from build123d import *

# Parameters (mm, degrees)
SKETCH1_R           = 3
BOSS_EXTRUDE1_DEPTH = 1.6


with BuildPart() as part:
    # Sketch1 → Boss-Extrude1 (new body)
    with BuildSketch(Plane(origin=(0, 0, 0), x_dir=(1, 0, 0), z_dir=(0, 1, 0))):
        with BuildLine():
            ThreePointArc((95.75, 0), (98.5, 2.75), (101.25, 0))
            Line((101.25, 0), (102, 0))
            Line((102, 0), (102, 11.75))
            ThreePointArc((102, 11.75), (113.75, 23.5), (125.5, 11.75))
            Line((125.5, 11.75), (125.5, 0))
            Line((125.5, 0), (126.25, 0))
            ThreePointArc((126.25, 0), (129, 2.75), (131.75, 0))
            Line((131.75, 0), (145.25, 0))
            ThreePointArc((145.25, 0), (148, 2.75), (150.75, 0))
            Line((150.75, 0), (151.5, 0))
            Line((151.5, 0), (151.5, 11.75))
            ThreePointArc((151.5, 11.75), (163.25, 23.5), (175, 11.75))
            Line((175, 11.75), (175, 0))
            Line((175, 0), (175.75, 0))
            ThreePointArc((175.75, 0), (178.5, 2.75), (181.25, 0))
            Line((181.25, 0), (190, 0))
            Line((190, 0), (184.397294991, 13.35112683))
            ThreePointArc((184.397294991, 13.35112683), (175.255085608, 21.137460938), (176.103062866, 33.116105511))
            Line((176.103062866, 33.116105511), (166.5, 56))
            Line((166.5, 56), (162.25, 56))
            ThreePointArc((162.25, 56), (159.5, 53.25), (156.75, 56))
            Line((156.75, 56), (156, 56))
            Line((156, 56), (156, 44.25))
            ThreePointArc((156, 44.25), (144.25, 32.5), (132.5, 44.25))
            Line((132.5, 44.25), (132.5, 56))
            Line((132.5, 56), (131.75, 56))
            ThreePointArc((131.75, 56), (129, 53.25), (126.25, 56))
            Line((126.25, 56), (106.5, 56))
            Line((106.5, 56), (106.5, 44.25))
            ThreePointArc((106.5, 44.25), (94.75, 32.5), (83, 44.25))
            Line((83, 44.25), (83, 56))
            Line((83, 56), (35, 56))
            Line((35, 56), (28.772512455, 46.036019928))
            ThreePointArc((28.772512455, 46.036019928), (29.720282193, 45.037138056), (30.06501537, 43.704024592))
            ThreePointArc((30.06501537, 43.704024592), (28.648128834, 41.298757768), (25.857518285, 41.372029256))
            Line((25.857518285, 41.372029256), (23.160953678, 37.057525885))
            ThreePointArc((23.160953678, 37.057525885), (27.537926652, 32.444507786), (29.12996714, 26.287947424))
            ThreePointArc((29.12996714, 26.287947424), (22.586527501, 15.179987912), (9.698980602, 15.518368963))
            Line((9.698980602, 15.518368963), (8.612482775, 13.77997244))
            ThreePointArc((8.612482775, 13.77997244), (9.560252513, 12.781090568), (9.90498569, 11.447977104))
            ThreePointArc((9.90498569, 11.447977104), (8.488099154, 9.042710281), (5.697488605, 9.115981768))
            Line((5.697488605, 9.115981768), (0, 0))
            Line((0, 0), (95.75, 0))
        make_face()
        with Locations(Location((92, 11.75, 0), (0, 0, 270))):  # turned: the seam where the file's is
            Circle(SKETCH1_R, mode=Mode.SUBTRACT)
        with Locations(Location((73, 44.25, 0), (0, 0, 270))):  # turned: the seam where the file's is
            Circle(SKETCH1_R, mode=Mode.SUBTRACT)
        with Locations(Location((122.5, 44.25, 0), (0, 0, 270))):  # turned: the seam where the file's is
            Circle(SKETCH1_R, mode=Mode.SUBTRACT)
    extrude(amount=BOSS_EXTRUDE1_DEPTH)


solid = part.part
Verification items for the finished model (mm, model axes). Coordinates: 2 decimals unless noted, no trailing zeros. Order: outer loops, then holes, each group sorted by start corner. A loop starts at its lowest first (then second) coordinate and runs counter-clockwise, first axis right, second up. Notation, with made-up numbers: M 20,-34 L 38,-34 A13 ccw 38,-14 Z; hole C 83,67.5 d2. An arc over 180 degrees is marked long. Write each question's results on one line, items separated by ' | '.
1) Release check for a two-part mould opening along Z. For faces 1 (the face through (89.07, 0.79, -12.4)), 2 (the face through (94, 0, -28)), 3 (the face through (125.474, 0.789, -44.641)), 4 (the face through (187.24, 0.79, -6.58)) record: pulls with the +Z half, pulls with the -Z half, needs draft (parallel to the pull), parting line crosses it, or undercut.
Solved:
face 1: undercut | face 2: needs draft | face 3: undercut | face 4: pulls with the -Z half
2) Scan lines: line 1 along X through (y, z) = (1.15, -37); line 2 along X through (y, z) = (0.1, -44); line 3 along X through (y, z) = (0.35, -3.5). Record each from-to range of solid material in increasing order. Write a range as [from, to].
Solved:
line 1: x = [23.25, 85.5], [104, 135], [153.5, 174.47] | line 2: x = [30.05, 70.01], [75.99, 83], [106.5, 119.51], [125.49, 132.5], [156, 171.54] | line 3: x = [2.19, 102], [125.5, 151.5], [175, 188.53]
3) Gauge pin test, flat ends, axial feed: pin 1 Ø4 at (x, z) = (69, -11.5) entering from -Y; pin 2 Ø0.8 at (y, z) = (1, -3) entering from -X (3 decimals); pin 3 Ø0.8 at (y, z) = (0.5, -49.5) entering from +X; pin 4 Ø0.5 at (y, z) = (0.5, -49) entering from -X. Record the tip position at first contact, or that the pin passes through.
Solved:
pin 1: stops at y = 0 | pin 2: stops at x = 1.625 | pin 3: stops at x = 169.4 | pin 4: stops at x = 30.47
4) Section check A-A on x = 73. Record the cut outline in (y, z).
Solved:
outline: M 0,-56 L 1.6,-56 L 1.6,-47.25 L 0,-47.25 Z; M 0,-41.25 L 1.6,-41.25 L 1.6,0 L 0,0 Z
5) Section check B-B on z = -50.5. Record the cut outline in (x, y).
Solved:
outline: M 31.56,0 L 83,0 L 83,1.6 L 31.56,1.6 Z; M 106.5,0 L 132.5,0 L 132.5,1.6 L 106.5,1.6 Z; M 156,0 L 168.81,0 L 168.81,1.6 L 156,1.6 Z
6) Section check C-C on y = 0.45. Give the number of separate pieces and of enclosed holes in the cut face, plus the area to 3 significant figures.
Solved:
separate pieces: 1 | enclosed holes: 3 | area: 6,520 mm²
7) Section check D-D on x = 122.5. Record the cut outline in (y, z), plus the area to 3 significant figures.
Solved:
outline: M 0,-56 L 1.6,-56 L 1.6,-47.25 L 0,-47.25 Z; M 0,-41.25 L 1.6,-41.25 L 1.6,-19.59 L 0,-19.59 Z | area: 48.7 mm²
